Autodesk Inventor part; units mm, degrees
ref_plane "YZ Plane" through (0, 0, 0) normal (1, 0, 0) x (0, 1, 0)
ref_plane "XZ Plane" through (0, 0, 0) normal (0, 1, 0) x (-1, 0, 0)
ref_plane "XY Plane" through (0, 0, 0) normal (0, 0, 1) x (1, 0, 0)
sketch "Sketch1" plane through (0, 0, 0) normal (0, 0, 1) x (1, 0, 0)
  line L0 (0, 3.048) -> (-43.4864, 3.048) construction
  line L1 (-43.4864, 0) -> (-43.4864, 3.048)
  line L2 (-43.4864, 0) -> (0, 0)
  line L3 (0, 0) -> (0, 3.048)
  line L4 (0, 88.646) -> (-43.4864, 88.646)
  line L5 (-43.4864, 85.598) -> (-43.4864, 88.646)
  line L6 (-43.4864, 85.598) -> (0, 85.598) construction
  line L7 (0, 85.598) -> (0, 88.646)
  line L8 (0, 0) -> (-43.4864, 0)
  line L9 (-43.4864, 0) -> (-43.4864, 88.646)
  line L10 (-43.4864, 88.646) -> (0, 88.646)
  line L11 (0, 88.646) -> (0, 0)
extrude "Plate1" add sketch "Sketch1" along normal blind 3.048
sketch "Sketch2" plane through (-43.4864, 0, 0) normal (0, -1, 0) x (1, 0, 0)
  line L0 (43.4864, 0) -> (0, 0)
  line L1 (0, 0) -> (0, -200.152)
  line L2 (0, -200.152) -> (43.4864, -200.152)
  line L3 (43.4864, -200.152) -> (43.4864, 0)
edge flange "Flange1" height 203.2 angle 90 thickness 3.048 bend radius 3.048 thickness toward (0, -1, 0) relief tear relief width 3.048 relief depth 1.524 corner gap 3.048 corner form 0 edges at (-21.7432, 0, 0) (-21.7432, 88.646, 0) wall of the first edge with corners at (0, 0, 0) (-43.4864, 0, 0) (-43.4864, 0, -200.152) (0, 0, -200.152)
bend "Bend1"
corner "Corner1"
sketch "Sketch3" plane through (0, 0, 3.048) normal (0, 0, 1) x (1, 0, 0)
  line L0 (-43.4864, 3.048) -> (-43.4864, 15.748) construction
  line L1 (-43.4864, 15.748) -> (-21.8429, 38.5703)
  line L2 (-16.3873, 44.323) -> (-20.9038, 49.0855) construction
  line L3 (-43.4864, 85.598) -> (-43.4864, 72.898) construction
  line L4 (-43.4864, 3.048) -> (-43.4864, 85.598)
  line L5 (-43.4864, 72.898) -> (-43.4864, 15.748)
  line L6 (-19.5391, 49.0855) -> (-14.5538, 49.0855)
  line L7 (-11.3788, 45.9105) -> (-11.3788, 42.7355)
  line L8 (-14.5538, 39.5605) -> (-19.5391, 39.5605)
  line L9 (-20.9038, 39.5605) -> (-16.3873, 44.323) construction
  line L10 (-21.8429, 50.0757) -> (-43.4864, 72.898)
  arc A0 (-14.5538, 39.5605) -> (-11.3788, 42.7355) centre (-14.5538, 42.7355) ccw
  arc A1 (-11.3788, 45.9105) -> (-14.5538, 49.0855) centre (-14.5538, 45.9105) ccw
  arc A2 (-21.8429, 50.0757) -> (-19.5391, 49.0855) centre (-19.5391, 52.2605) ccw
  arc A3 (-19.5391, 39.5605) -> (-21.8429, 38.5703) centre (-19.5391, 36.3855) ccw
  line L11 (-43.4864, 3.048) -> (-43.4864, 85.598)
  point P0 (0, 0)
  point P1 (-11.3788, 49.0855)
  point P2 (-11.3788, 39.5605)
  dimension "d11" = 12.7
  dimension "d12" = 28.575
  dimension "d14" = 12.7
  dimension "d18" = 9.525
  dimension "d19" = 9.525
  dimension "d20" = 9.525
  dimension "d24" = 3.175
  dimension "d25" = 11.5054
extrude "Extrusion1" cut sketch "Sketch3" against normal up to next
sketch "Sketch4" plane through (-43.4864, -3.048, -200.152) normal (0, -1, 0) x (1, 0, 0)
  circle A0 centre (12.7, 6.35) radius 2.54
  circle A1 centre (30.7864, 6.35) radius 2.54
  line L0 (0, 0) -> (0, 197.104)
  line L1 (43.4864, 0) -> (0, 0)
  line L2 (43.4864, 0) -> (43.4864, 197.104)
  point P0 (43.4864, 200.152)
  dimension "d26" = 5.08
  dimension "d27" = 5.08
  dimension "d28" = 12.7
  dimension "d29" = 6.35
  dimension "d30" = 6.35
  dimension "d31" = 12.7
extrude "Extrusion2" cut sketch "Sketch4" against normal up to surface (94.742 mm away)
equation "\"d1\" = BendReliefWidth"
equation "\"d2\" = BendReliefDepth"
equation "\"d3\" = MinimumRemnant"
equation "\"d4\" = BendRadius"
equation "\"d7\" = BendRadius"
equation "\"d8\" = CornerReliefSize"
equation "\"d9\" = GapSize"
equation "\"d10\" = JacobiRadiusSize"
equation "\"BendRadius\" = Thickness"
equation "\"BendReliefWidth\" = Thickness"
equation "\"BendReliefDepth\" = 0.5 * Thickness"
equation "\"CornerReliefSize\" = 4 * Thickness"
equation "\"MinimumRemnant\" = 2 * Thickness"
equation "\"TransitionRadius\" = BendRadius"
equation "\"JacobiRadiusSize\" = BendRadius"
equation "\"GapSize\" = Thickness"
equation "\"d0\" = BendRadius"
properties part number "guidebar"
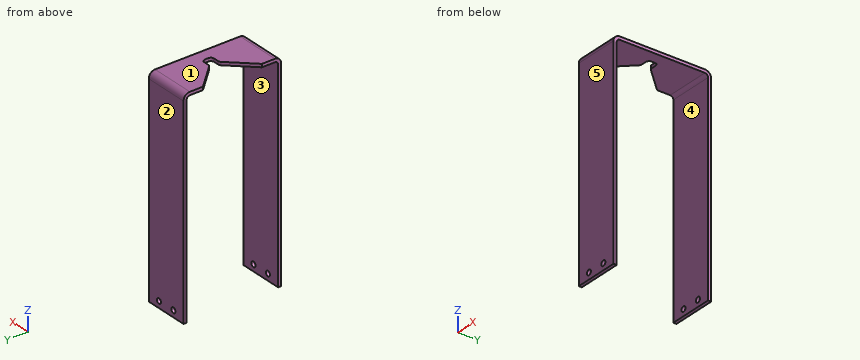
Here's how the part is built. I have some questions about the finished solid (model axes, mm). Face numbers are marked on the shaded views. A direction names the side the tool comes from. Give positions to 0.01 mm unless a question says otherwise; leave off trailing zeros. Loops run counter-clockwise (first coordinate to the right, second up) from the corner with the lowest first, then second, coordinate; pieces in that order, holes last. Notation, with made-up numbers: M 83,-29.5 L 91,-29.5 A18 ccw 91,-13.5 Z; hole C -38.75,11.25 d5. An arc over 180 degrees is marked long. Use one line per item in the form item = value. Start each with the question number.
Q1. Which directions (+Z, -Z, +X, -X, +Y, -Y) give clear straight access to the entire face, cutting with the end or side of a thin tool? Please do the marked faces 4 and 5.
Q2. If we section it at D-D (y = 11): Write out the boundary of the cut face in (x, z), then the cut area to 3 significant figures.
Q3. If we section it at A-A (z = -40): Write out the boundary of the cut face in (x, y).
Q4. Thinking about a two-plate mould opening in Y: for the marked faces 1, 2 and 3, which applies, +Y half, -Y half, draft (parallel to the pull), parting line (faces both ways), or undercut?
Q5. Will these pins go through, and if not, where does the flat tip stop? pin 1 Ø3 at (x, y) = (-12.5, 42) entering from -Z; pin 2 Ø2.5 at (y, z) = (45, 1) entering from -X; pin 3 Ø1.5 at (x, z) = (-17, 1) entering from -Y.
Q6. If we section it at B-B (x = -25): Write out the boundary of the cut face in (y, z), then the cut area to 3 significant figures.
Q7. If we section it at C-C (x = -40): Write out the boundary of the cut face in (y, z).
Q8. I need wall thicknesses on line 1 along Y through (x, z) = (-11.5, -133); line 2 along Z through (x, y) = (-6.5, 41); line 3 along Z through (x, y) = (-12.7, 89.55). Which ranges of each line are inside material? Lowest first, please.
Taken from the geometry:
q1.face_4 = -Z, +X, -X
q1.face_5 = +Z, -Z, +X, -X, -Y
q2.outline = M -43.49,0 L 0,0 L 0,3.05 L -43.49,3.05 Z
q2.area = 133 mm^2
q3.outline = M -43.49,-3.05 L 0,-3.05 L 0,0 L -43.49,0 Z; M -43.49,88.65 L 0,88.65 L 0,91.69 L -43.49,91.69 Z
q4.face_1 = draft
q4.face_2 = +Y half
q4.face_3 = undercut
q5.pin_1 = 0
q5.pin_2 = -11.4
q5.pin_3 = -2.08
q6.outline = M -3.05,-200.15 L 0,-200.15 L 0,-3.05 A3.05 cw 3.05,0 L 35.24,0 L 35.24,3.05 L 3.05,3.05 A6.1 ccw -3.05,-3.05 Z; M 53.4,0 L 85.6,0 A3.05 cw 88.65,-3.05 L 88.65,-200.15 L 91.69,-200.15 L 91.69,-3.05 A6.1 ccw 85.6,3.05 L 53.4,3.05 Z
q6.area = 1,440 mm^2
q7.outline = M -3.05,-200.15 L 0,-200.15 L 0,-3.05 A3.05 cw 3.05,0 L 19.42,0 L 19.42,3.05 L 3.05,3.05 A6.1 ccw -3.05,-3.05 Z; M 69.22,0 L 85.6,0 A3.05 cw 88.65,-3.05 L 88.65,-200.15 L 91.69,-200.15 L 91.69,-3.05 A6.1 ccw 85.6,3.05 L 69.22,3.05 Z
q8.line_1 = -3.05 to 0, 88.65 to 91.69
q8.line_2 = 0 to 3.05
q8.line_3 = -200.15 to -196.34, -191.26 to 1.59
